Model file for the job. Use its own axes, mm. A direction names the side the tool comes from. Coordinates: 2 decimals unless noted, no trailing zeros. Loops run counter-clockwise (first coordinate to the right, second up) from the corner with the lowest first, then second, coordinate; pieces in that order, holes last.
Autodesk Inventor part; units mm, degrees
ref_plane "YZ Plane" through (0, 0, 0) normal (1, 0, 0) x (0, 1, 0)
ref_plane "XZ Plane" through (0, 0, 0) normal (0, 1, 0) x (-1, 0, 0)
ref_plane "XY Plane" through (0, 0, 0) normal (0, 0, 1) x (1, 0, 0)
sketch "Sketch1" plane through (0, 0, 0) normal (0, 1, 0) x (-1, 0, 0)
  line L0 (0, -16) -> (0, 0)
  line L1 (0, 0) -> (-66, 0)
  line L2 (-66, 0) -> (-66, -16)
  line L3 (-66, -16) -> (-41, -16)
  line L4 (-41, -16) -> (-41, -36)
  line L5 (-41, -36) -> (-25, -36)
  line L6 (-25, -36) -> (-25, -16)
  line L7 (-25, -16) -> (0, -16)
  circle A0 centre (-8, -8) radius 2.25
  circle A1 centre (-58, -8) radius 2.25
  line L8 (-35.3094, -24) -> (-30.6906, -24)
  line L9 (-30.6906, -24) -> (-28.3812, -28)
  line L10 (-28.3812, -28) -> (-30.6906, -32)
  line L11 (-30.6906, -32) -> (-35.3094, -32)
  line L12 (-35.3094, -32) -> (-37.6188, -28)
  line L13 (-37.6188, -28) -> (-35.3094, -24)
  point P0 (0, -8)
  point P1 (-33, -28)
  point P2 (-33, -36)
  dimension "d0" = 16
  dimension "d1" = 4.5
  dimension "d2" = 50
  dimension "d3" = 8
  dimension "d4" = 8
  dimension "d5" = 16
  dimension "d6" = 36
  dimension "d7" = 8
  dimension "d8" = 20
extrude "Extrusion1" add sketch "Sketch1" along normal blind 6.5
chamfer "Chamfer1" distance 4 angle 45 8 edges at (66, 3.25, 0) (66, 3.25, -16) (0, 3.25, 0) (0, 3.25, -16) (25, 3.25, -16) (25, 3.25, -36) (41, 3.25, -36) (41, 3.25, -16)
equation "\"d3\" = 0.5 * d0"
equation "\"d4\" = d3"
properties part number "y_carriage_nut_holder_b" material "Plywood, Finish"
Q1. Flat gauge pins, fed straight in: P1, Ø2, axis at x = 55.5, y = 4, coming from the -Z side; P2, Ø1, axis at x = 24.5, z = -20, coming from the +Y side; P3, Ø3, axis at y = 5, z = -26, coming from the -X side. Where does each tip first touch, or does it go through?
Answers:
P1: stops at z = -16
P2: stops at y = 6.5
P3: stops at x = 25
Q2. Slice it at D-D (z = -31). List the corners of the cut face in (x, y).
Answers:
outline: (25, 0) - (30.11, 0) - (30.11, 6.5) - (25, 6.5) - close; (35.89, 0) - (41, 0) - (41, 6.5) - (35.89, 6.5) - close
Q3. Slice it at C-C (y = 0.75). List the corners of the cut face in (x, z).
Answers:
outline: (0, -12) - (4, -16) - (21, -16) - (25, -20) - (25, -32) - (29, -36) - (37, -36) - (41, -32) - (41, -20) - (45, -16) - (62, -16) - (66, -12) - (66, -4) - (62, 0) - (4, 0) - (0, -4) - close; hole circle Ø4.5 at (8, -8); hole (28.38, -28) - (30.69, -32) - (35.31, -32) - (37.62, -28) - (35.31, -24) - (30.69, -24) - close; hole circle Ø4.5 at (58, -8)
Q4. Mould opens along X. For faces 1 (the flat face through (36.48, 3.2, -26.03)), 2 (the flat face through (25, 3, -26)), 3 (the flat face through (54, 3, -16)) say: +X half, -X half, draft (parallel to the pull), parting line (faces both ways), or undercut.
Answers:
face 1: undercut
face 2: -X half
face 3: draft
Q5. Which spindle directions (+Z, -Z, +X, -X, +Y, -Y) get a long thin tool onto all of the face, cutting with end or side? Do faces 4 (the flat face through (29.552, 3.204, -25.972)), 5 (the flat face through (33, 6.5, -10)), 6 (the flat face through (41, 3, -26)). Say none if no direction does.
Answers:
face 4: +Y, -Y
face 5: +Z, -Z, +X, -X, +Y
face 6: -Z, +X, +Y, -Y
Q6. Drill centre lines: line 1 (Z direction, x = 58, y = 4.5); line 2 (X direction, y = 3.25, z = -7); line 3 (X direction, y = 5, z = -28). Where is each one in solid material? Low to high.
Answers:
line 1: z = -16 to -10.25, -5.75 to 0
line 2: x = 0 to 5.98, 10.02 to 55.98, 60.02 to 66
line 3: x = 25 to 28.38, 37.62 to 41
Q7. Slice it at B-B (x = 8). List the corners of the cut face in (y, z).
Answers:
outline: (0, -16) - (6.5, -16) - (6.5, -10.25) - (0, -10.25) - close; (0, -5.75) - (6.5, -5.75) - (6.5, 0) - (0, 0) - close
Q8. Slice it at A-A (z = -8). List the corners of the cut face in (x, y).
Answers:
outline: (0, 0) - (5.75, 0) - (5.75, 6.5) - (0, 6.5) - close; (10.25, 0) - (55.75, 0) - (55.75, 6.5) - (10.25, 6.5) - close; (60.25, 0) - (66, 0) - (66, 6.5) - (60.25, 6.5) - close
